Part model, mm, in its own coordinate system. A direction names the side the tool comes from. Coordinates: 2 decimals unless noted, no trailing zeros. Write each loop counter-clockwise with the first axis right and the second up, starting at its lowest first coordinate (ties: lowest second). Pieces come first, ordered by that corner, then holes. Notation, with made-up numbers: (-9, 17.5) - (-5, 17.5) arc R22 ccw to (-5, 28.5) - close; hole circle Ø10 at (38.5, -17.5). An arc over 180 degrees is marked (long way). Use a Markdown table: item, result.
Autodesk Inventor part; units mm, degrees
ref_plane "YZ Plane" through (0, 0, 0) normal (1, 0, 0) x (0, 1, 0)
ref_plane "XZ Plane" through (0, 0, 0) normal (0, 1, 0) x (-1, 0, 0)
ref_plane "XY Plane" through (0, 0, 0) normal (0, 0, 1) x (1, 0, 0)
sketch "Sketch1" plane through (0, 0, 0) normal (0, 0, 1) x (1, 0, 0)
  line L0 (0, 0) -> (41.7159, 0)
  line L1 (41.7159, 0) -> (41.7159, 6)
  line L2 (41.7159, 6) -> (0, 6)
  line L3 (0, 6) -> (0, 0)
  line L4 (0, 6) -> (41.7159, 35.2098)
  line L5 (41.7159, 6) -> (41.7159, 35.2098)
  circle A0 centre (31.7159, 16) radius 10
  point P0 (41.7159, 16)
  point P1 (25.9802, 24.1915)
  dimension "d0" = 35
  dimension "d1" = 6
  dimension "d12" = 20
extrude "Extrusion1" add sketch "Sketch1" along normal blind 10 contours L3 L2 L1 L0 | L4 A0 L2 | L2 A0 L5 | A0
sketch "Sketch3" plane through (0, 0, 0) normal (0, 0, -1) x (-1, 0, 0)
  line L0 (-41.7159, 0) -> (-41.7159, 16)
  line L1 (0, 0) -> (-41.7159, 0)
  line L2 (0, 6) -> (0, 0)
  line L3 (-25.9802, 24.1915) -> (0, 6)
  line L4 (-47.336, 39.1451) -> (0, 6)
  line L5 (-41.7159, 0) -> (0, 0)
  line L6 (0, 0) -> (0, 6)
  line L7 (0, 6) -> (-41.7159, 6)
  line L8 (-41.7159, 6) -> (-41.7159, 0)
  arc A0 (-25.9802, 24.1915) -> (-41.7159, 16) centre (-31.7159, 16) ccw
  point P0 (-46.3964, 40.4871)
extrude "Extrusion3" add sketch "Sketch3" along normal blind 10 contours L0 L7 L2 L1
sketch "Sketch4" plane through (0, 0, 10) normal (0, 0, 1) x (1, 0, 0)
  line L0 (0, 6) -> (0, 0)
  line L1 (0, 0) -> (41.7159, 0)
  line L2 (41.7159, 0) -> (41.7159, 16)
  arc A0 (41.7159, 16) -> (25.9802, 24.1915) centre (31.7159, 16) ccw
  line L3 (25.9802, 24.1915) -> (0, 6)
  line L4 (31.7159, 26) -> (50, 26)
  line L5 (50, 26) -> (50, 0)
  line L6 (50, 0) -> (31.7159, 0)
  line L7 (31.7159, 0) -> (31.7159, 26)
  arc A1 (41.7159, 16) -> (25.9802, 24.1915) centre (31.7159, 16) ccw
  point P0 (41.7159, 0)
  dimension "d14" = 50
extrude "Extrusion4" add sketch "Sketch4" against normal up to surface (10 mm away) contours L4 L5 L6 L2 A0
sketch "Sketch5" plane through (41.7159, 0, 0) normal (1, 0, 0) x (0, 0, -1)
  line L0 (0, 6) -> (0, 0)
  line L1 (0, 0) -> (10, 0)
  line L2 (10, 6) -> (10, 0)
  line L3 (0, 6) -> (10, 6)
  point P0 (0, 0)
extrude "Extrusion5" add sketch "Sketch5" along normal up to surface (8.2841 mm away)
properties part number "Print_Parts_F1"
Item 1: Drill centre lines: probe 1 along Y at (x, z) = (40, -5.75); probe 2 along Z at (x, y) = (17.5, 15.75); probe 3 along X at (y, z) = (17.75, 2.5). Where is each one in solid material? Low to high.
From the geometry:
| item | result |
|---|---|
| probe 1 | 0 to 6 |
| probe 2 | 0 to 10 |
| probe 3 | 16.78 to 50 |
Item 2: Band-saw the part on B-B, the plane z = 1.5. Give the cut face in (x, y), then the cut area to 3 significant figures.
From the geometry:
| item | result |
|---|---|
| outline | (0, 0) - (50, 0) - (50, 26) - (31.72, 26) arc R10 ccw to (25.98, 24.19) - (0, 6) - close |
| area | 1,010 mm^2 |
Item 3: Band-saw the part on D-D, the plane z = -2.5. Give the cut face in (x, y).
From the geometry:
| item | result |
|---|---|
| outline | (0, 0) - (50, 0) - (50, 6) - (0, 6) - close |
Item 4: Band-saw the part on A-A, the plane x = 44. Give the cut face in (y, z).
From the geometry:
| item | result |
|---|---|
| outline | (0, -10) - (6, -10) - (6, 0) - (26, 0) - (26, 10) - (0, 10) - close |
Item 5: Two-plate mould, pull along Y, no slides. Class faces 1 (the face through (25, 0, 0)), 2 (the face through (0, 3, 0)), 3 (the face through (41, 26, 5)): pulls with the +Y half, pulls with the -Y half, needs draft (parallel to the pull), parting line crosses it, or undercut.
From the geometry:
| item | result |
|---|---|
| face 1 | pulls with the -Y half |
| face 2 | needs draft |
| face 3 | pulls with the +Y half |
Item 6: Which spindle directions (+Z, -Z, +X, -X, +Y, -Y) get a long thin tool onto all of the face, cutting with end or side? Do faces 4 (the face through (30, 14, 0)), 5 (the face through (28.668, 25.524, 4.93)). Say none if no direction does.
From the geometry:
| item | result |
|---|---|
| face 4 | -Z, +X, -X, +Y |
| face 5 | +Z, -Z, -X, +Y |
Item 7: Drop flat-ended pins along their axis: P1, Ø10, axis at x = 19.5, y = 14.5, coming from the -Z side; P2, Ø4, axis at x = 8, z = 1, coming from the +Y side; P3, Ø3, axis at x = 17.5, z = -4, coming from the +Y side; P4, Ø10, axis at y = 14, z = -5.5, coming from the +X side. Give the stop position or say it passes through.
From the geometry:
| item | result |
|---|---|
| P1 | z = 0 |
| P2 | y = 13 |
| P3 | y = 6 |
| P4 | through |
Item 8: Band-saw the part on C-C, the plane y = 22. Give the cut face in (x, z).
From the geometry:
| item | result |
|---|---|
| outline | (22.85, 0) - (50, 0) - (50, 10) - (22.85, 10) - close |
